For this review, take the finished solid that the model builds, in its own axes (mm). Face numbers are marked on the shaded views. A direction names the side the tool comes from. Give positions to 0.01 mm unless a question says otherwise; leave off trailing zeros. Write each loop counter-clockwise with the first axis right and the second up, starting at its lowest first coordinate (ties: lowest second). Pieces come first, ordered by that corner, then holes. Notation, with made-up numbers: M 16,25 L 47,25 A16 ccw 47,46 Z; hole C 29.5,-28.5 d5. An arc over 180 degrees is marked long. Answer as a JSON object with one key per item and string values. Group by question number.
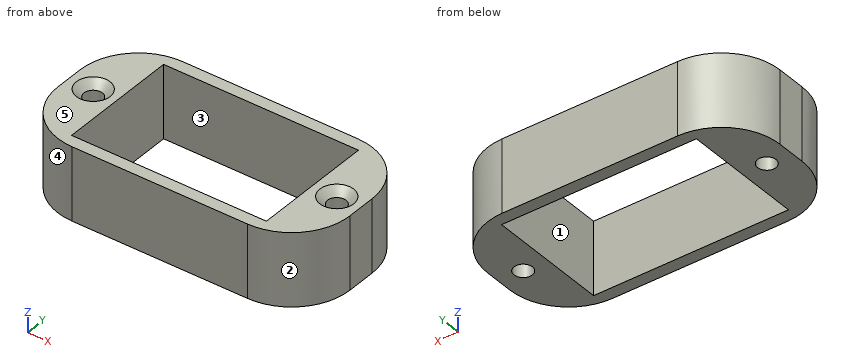
```python
from build123d import *

# Parameters (mm, degrees)
SKETCH1_W                                       = 38.1
SKETCH1_H                                       = 19.05
BOSS_EXTRUDE1_DEPTH                             = 9.525
SKETCH2_W                                       = 25.4
SKETCH2_H                                       = 15.875
CUT_EXTRUDE1_DEPTH                              = 9.525
FILLET1_R                                       = 7.62
CSK_FOR_M2_FLAT_HEAD_MACHINE_SCREW1_D           = 2.4
CSK_FOR_M2_FLAT_HEAD_MACHINE_SCREW1_CSINK_D     = 4.4
CSK_FOR_M2_FLAT_HEAD_MACHINE_SCREW1_CSINK_ANGLE = 90


with BuildPart() as part:
    # Sketch1 → Boss-Extrude1 (new body)
    with BuildSketch(Plane.XY):
        Rectangle(SKETCH1_W, SKETCH1_H)
    extrude(amount=BOSS_EXTRUDE1_DEPTH)

    # Sketch2 → Cut-Extrude1 (cut)
    with BuildSketch(Plane.XY.offset(9.525)):
        Rectangle(SKETCH2_W, SKETCH2_H)
    extrude(amount=-CUT_EXTRUDE1_DEPTH, mode=Mode.SUBTRACT)

    # Fillet1
    fillet1_edges = [part.edges().sort_by_distance(p)[0] for p in [
        (-19.05, 9.525, 4.7625),
        (19.05, 9.525, 4.7625),
        (19.05, -9.525, 4.7625),
        (-19.05, -9.525, 4.7625),
    ]]
    fillet(fillet1_edges, radius=FILLET1_R)

    # CSK for M2 Flat Head Machine Screw1 (through all)
    with Locations(Plane.XY.offset(9.525)):
        with Locations((-15.875, 0), (15.875, 0)):
            CounterSinkHole(CSK_FOR_M2_FLAT_HEAD_MACHINE_SCREW1_D / 2, CSK_FOR_M2_FLAT_HEAD_MACHINE_SCREW1_CSINK_D / 2, counter_sink_angle=CSK_FOR_M2_FLAT_HEAD_MACHINE_SCREW1_CSINK_ANGLE)


solid = part.part
```
Item 1: Machinability: for the marked faces 1 and 2, which of the approach directions +Z, -Z, +X, -X, +Y, -Y give a long, thin tool a straight path to every point of the face, cutting with its end or side? Answer none if there is none.
Item 2: Consider section B-B (z = 3). State how many separate pieces and enclosed holes the cut face has, plus the area to 3 significant figures.
Item 3: To check wall thickness, follow probe 1 along X at (y, z) = (0, 4.75) (3 decimals); probe 2 along X at (y, z) = (-1.75, 5.25); probe 3 along X at (y, z) = (-1, 4.75). State the ranges of each line that lie inside material, in increasing order.
Item 4: Draft analysis for pull direction X (two halves, no side actions). For the marked faces 3, 4 and 5, state which applies: released by +X, released by -X, zero draft, split by the parting line, or undercut.
Item 5: Consider section D-D (y = -4.5). Give the boundary of the cut face in (x, z) (3 decimals), plus the area to 3 significant figures.
Item 6: Insertion check: P1, Ø2, axis at x = 3.5, y = 5, coming from the -Z side; P2, Ø2, axis at y = 7, z = 3, coming from the -X side. Each pin has a flat end and moves straight along its axis. Give the tip position at first contact, or say it passes through.
Item 7: Consider section C-C (y = 0). Give the boundary of the cut face in (x, z) (3 decimals), plus the area to 3 significant figures.
Item 8: Consider section A-A (x = -10). Give the boundary of the cut face in (y, z) (1 decimal).
Result set:
{
 "1": {"face 1": "+Z, -Z", "face 2": "+Z, -Z, +X, -Y"},
 "2": {"separate pieces": "1", "enclosed holes": "3", "area": "264 mm^2"},
 "3": {"probe 1": "x = -19.05 to -17.075, -14.675 to -12.7, 12.7 to 14.675, 17.075 to 19.05", "probe 2": "x = -19.05 to -12.7, 12.7 to 19.05", "probe 3": "x = -19.05 to -16.54, -15.21 to -12.7, 12.7 to 15.21, 16.54 to 19.05"},
 "4": {"face 3": "undercut", "face 4": "released by -X", "face 5": "zero draft"},
 "5": {"outline": "M -18.595,0 L -12.7,0 L -12.7,9.525 L -18.595,9.525 Z; M 12.7,0 L 18.595,0 L 18.595,9.525 L 12.7,9.525 Z", "area": "112 mm^2"},
 "6": {"P1": "passes through", "P2": "stops at x = -17.86"},
 "7": {"outline": "M -19.05,0 L -17.075,0 L -17.075,8.525 L -18.075,9.525 L -19.05,9.525 Z; M -14.675,0 L -12.7,0 L -12.7,9.525 L -13.675,9.525 L -14.675,8.525 Z; M 12.7,0 L 14.675,0 L 14.675,8.525 L 13.675,9.525 L 12.7,9.525 Z; M 17.075,0 L 19.05,0 L 19.05,9.525 L 18.075,9.525 L 17.075,8.525 Z", "area": "73.2 mm^2"},
 "8": {"outline": "M -9.5,0 L -7.9,0 L -7.9,9.5 L -9.5,9.5 Z; M 7.9,0 L 9.5,0 L 9.5,9.5 L 7.9,9.5 Z"}
}
